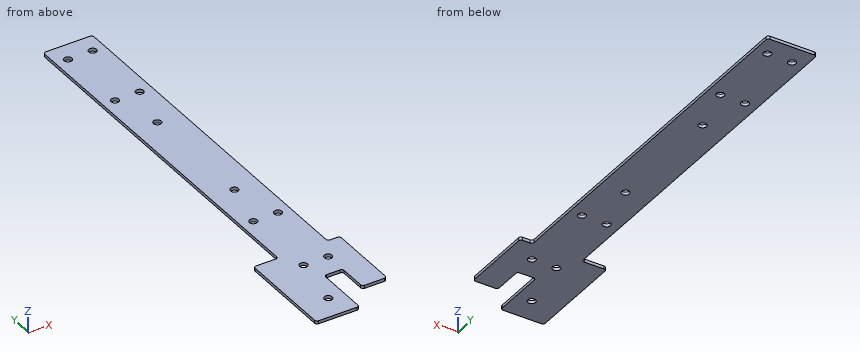
```python
from build123d import *

# Parameters (mm, degrees)
BOSS_EXTRUDE1_OUTLINE_R = 3.96875
BOSS_EXTRUDE1_DEPTH     = 3.175
FILLET2_R               = 2.54


# Read off the part's stored shape, not the designer's step: Boss-Extrude1
with BuildPart() as part:
    # Boss-Extrude1 outline → Boss-Extrude1 (new body)
    with BuildSketch(Plane.XY):
        Polygon((25.4, 0), (-25.4, 0), (-25.4, -381), (-50.8, -381), (-50.8, -482.6), (-6.35, -482.6), (-6.35, -425.45), (12.7, -425.45), (12.7, -457.2), (38.1, -457.2), (38.1, -381), (25.4, -381), align=None)
        with Locations((-22.225, -457.2)):
            Circle(BOSS_EXTRUDE1_OUTLINE_R, mode=Mode.SUBTRACT)
        with Locations((-12.7, -402.082)):
            Circle(BOSS_EXTRUDE1_OUTLINE_R, mode=Mode.SUBTRACT)
        with Locations((-12.7, -320.675)):
            Circle(BOSS_EXTRUDE1_OUTLINE_R, mode=Mode.SUBTRACT)
        with Locations((12.7, -402.082)):
            Circle(BOSS_EXTRUDE1_OUTLINE_R, mode=Mode.SUBTRACT)
        with Locations((12.7, -320.675)):
            Circle(BOSS_EXTRUDE1_OUTLINE_R, mode=Mode.SUBTRACT)
        with Locations((0, -270.0655)):
            Circle(BOSS_EXTRUDE1_OUTLINE_R, mode=Mode.SUBTRACT)
        with Locations((-12.7, -96.52)):
            Circle(BOSS_EXTRUDE1_OUTLINE_R, mode=Mode.SUBTRACT)
        with Locations((-12.7, -20.32)):
            Circle(BOSS_EXTRUDE1_OUTLINE_R, mode=Mode.SUBTRACT)
        with Locations((0, -145.0975)):
            Circle(BOSS_EXTRUDE1_OUTLINE_R, mode=Mode.SUBTRACT)
        with Locations((12.7, -96.52)):
            Circle(BOSS_EXTRUDE1_OUTLINE_R, mode=Mode.SUBTRACT)
        with Locations((12.7, -20.32)):
            Circle(BOSS_EXTRUDE1_OUTLINE_R, mode=Mode.SUBTRACT)
    extrude(amount=BOSS_EXTRUDE1_DEPTH)

    # Fillet2
    fillet2_edges = [part.edges().sort_by_distance(p)[0] for p in [
        (25.4, 0, 1.5875),
        (25.4, -381, 1.5875),
        (38.1, -381, 1.5875),
        (38.1, -457.2, 1.5875),
        (12.7, -457.2, 1.5875),
        (12.7, -425.45, 1.5875),
        (-6.35, -425.45, 1.5875),
        (-6.35, -482.6, 1.5875),
        (-50.8, -482.6, 1.5875),
        (-50.8, -381, 1.5875),
        (-25.4, -381, 1.5875),
        (-25.4, 0, 1.5875),
    ]]
    fillet(fillet2_edges, radius=FILLET2_R)


solid = part.part
```
Design review of the part built by this model. Coordinates are the model's own, in mm. Coordinates: 2 decimals unless noted, no trailing zeros. Order: outer loops, then holes, each group sorted by start corner. A loop starts at its lowest first (then second) coordinate and runs counter-clockwise, first axis right, second up. Notation, with made-up numbers: M 45.25,-14 L 64.25,-14 A16 cw 64.25,-7 Z; hole C 18,28.5 d11. An arc over 180 degrees is marked long. Answer as a JSON object with one key per item and string values. Group by question number.
1) Add section B-B, the plane x = -42. Write out the cut boundary in (y, z) (3 decimals).
2) Wall thickness on L1, parallel to Y at x = -12.7, z = 2; L2, parallel to Y at x = 13.5, z = 0.25; L3, parallel to X at y = -401.5, z = 1.55: over which ranges is each line inside the solid? List them lowest first.
3) Add section D-D, the plane z = 2.2. Count the separate pieces of the cut face and the enclosed holes in it, then the cut area to 3 significant figures.
4) Add section C-C, the plane y = -192. Write out the cut boundary in (x, z) (3 decimals).
5) For pin 1 (9 mm diameter, centred on x = -22.225, y = -457.2, fed in from -Z); pin 2 (6.5 mm diameter, centred on x = 0, y = -270.07, fed in from +Z); pin 3 (1.6 mm diameter, centred on y = -161.5, z = 1, fed in from -X); pin 4 (1 mm diameter, centred on x = -38.5, z = 1.5, fed in from +Y), all flat-tipped, find the tip position at first contact; note any pin that passes through.
6) Add section A-A, the plane y = -96.52. Write out the cut boundary in (x, z) (3 decimals), then the cut area to 3 significant figures.
Computed values:
{
 "1": {"outline": "M -482.6,0 L -381,0 L -381,3.175 L -482.6,3.175 Z"},
 "2": {"L1": "y = -482.6 to -406.05, -398.11 to -324.64, -316.71 to -100.49, -92.55 to -24.29, -16.35 to 0", "L2": "y = -456.51 to -405.97, -398.19 to -324.56, -316.79 to -100.41, -92.63 to -24.21, -16.43 to 0", "L3": "x = -50.8 to -16.63, -8.77 to 8.77, 16.63 to 38.1"},
 "3": {"separate pieces": "1", "enclosed holes": "11", "area": "26,100 mm^2"},
 "4": {"outline": "M -25.4,0 L 25.4,0 L 25.4,3.175 L -25.4,3.175 Z"},
 "5": {"pin 1": "stops at z = 0", "pin 2": "passes through", "pin 3": "stops at x = -25.4", "pin 4": "stops at y = -381"},
 "6": {"outline": "M -25.4,0 L -16.669,0 L -16.669,3.175 L -25.4,3.175 Z; M -8.731,0 L 8.731,0 L 8.731,3.175 L -8.731,3.175 Z; M 16.669,0 L 25.4,0 L 25.4,3.175 L 16.669,3.175 Z", "area": "111 mm^2"}
}
